The model under review builds one solid part; all positions refer to its coordinate system, in mm. A direction names the side the tool comes from. Give positions to 0.01 mm unless a question says otherwise; leave off trailing zeros. Order: outer loops, then holes, each group sorted by start corner. A loop starts at its lowest first (then second) coordinate and runs counter-clockwise, first axis right, second up. Notation, with made-up numbers: (32, 70) - (38, 70) arc R19 cw to (38, 91) - close; hole circle Ø7 at (-30.5, 46.25). An arc over 180 degrees is marked (long way). Put each result on its own line as item: value.
```python
from build123d import *

# Parameters (mm, degrees)
F0_W     = 23.6
F0_H     = 28.4
F1_DEPTH = 20
F2_W     = 23.6
F2_H     = 1.31
F3_DEPTH = 13.5
F2_R     = 5.025
F4_DEPTH = 20.001


with BuildPart() as f1:
    # F0 (on Top) → F1 (new body)
    with BuildSketch(Plane.XY):
        Rectangle(F0_W, F0_H)
    extrude(amount=F1_DEPTH)

    # F2 (on face) → F3 (cut)
    with BuildSketch(Plane.XY.offset(20)):
        with Locations((0, 5.545)):
            Rectangle(F2_W, F2_H)
    extrude(amount=-F3_DEPTH, mode=Mode.SUBTRACT)

    # F2 (on face) → F4 (cut, through all)
    with BuildSketch(Plane.XY.offset(20)):
        with Locations((0, -5.7)):
            Circle(F2_R)
    extrude(amount=-F4_DEPTH, mode=Mode.SUBTRACT)


solid = f1.part
```
(1) For faces 4 (the flat face through (0, 10, 20)), 5 (the flat face through (0, 4.89, 13)), list the 3-axis set-ups (+Z, -Z, +X, -X, +Y, -Y) from which the entire face can be reached by the end or side of a thin tool; tool diameter is ignored.
The answers:
face 4: +Z, +X, -X, +Y, -Y
face 5: +Z, +X, -X
(2) Take a section at D-D, the plane z = 4.25. Write out the cut boundary in (x, y) (3 decimals), then the cut area to 3 significant figures.
The answers:
outline: (-11.8, -14.2) - (11.8, -14.2) - (11.8, 14.2) - (-11.8, 14.2) - close; hole circle Ø10.05 at (0, -5.7)
area: 591 mm^2
(3) Take a section at A-A, the plane z = 9.5. Write out the cut boundary in (x, y) (3 decimals).
The answers:
outline: (-11.8, -14.2) - (11.8, -14.2) - (11.8, 4.89) - (-11.8, 4.89) - close; (-11.8, 6.2) - (11.8, 6.2) - (11.8, 14.2) - (-11.8, 14.2) - close; hole circle Ø10.05 at (0, -5.7)
(4) Take a section at C-C, the plane y = -5.7. Write out the cut boundary in (x, z) (3 decimals), then the cut area to 3 significant figures.
The answers:
outline: (-11.8, 0) - (-5.025, 0) - (-5.025, 20) - (-11.8, 20) - close; (5.025, 0) - (11.8, 0) - (11.8, 20) - (5.025, 20) - close
area: 271 mm^2
(5) Take a section at B-B, the plane x = 0. Write out the cut boundary in (y, z) (3 decimals).
The answers:
outline: (-14.2, 0) - (-10.725, 0) - (-10.725, 20) - (-14.2, 20) - close; (-0.675, 0) - (14.2, 0) - (14.2, 20) - (6.2, 20) - (6.2, 6.5) - (4.89, 6.5) - (4.89, 20) - (-0.675, 20) - close
(6) Wall thickness on L1, parallel to Y at x = 0, z = 12 (3 decimals); L2, parallel to X at y = -6, z = 15.25; L3, parallel to Y at x = 9.5, z = 13.75: over which ranges is each line inside the solid? List them lowest first.
The answers:
L1: -14.2 to -10.725, -0.675 to 4.89, 6.2 to 14.2
L2: -11.8 to -5.02, 5.02 to 11.8
L3: -14.2 to 4.89, 6.2 to 14.2
(7) The part is to be moulded in two halves that separate along Y. For faces 1 (the cylindrical face through (-0.654, -0.718, 10.14)), 2 (the flat face through (0, -14.2, 10)), 3 (the flat face through (11.8, 0, 10)), say which applies: pulls with the +Y half, pulls with the -Y half, needs draft (parallel to the pull), parting line crosses it, or undercut.
The answers:
face 1: undercut
face 2: pulls with the -Y half
face 3: needs draft
